Answer from the drawing. Dimensions are ordinates in mm from the lowest x, y and z of the part. A direction names the side the tool comes from. Give positions to 0.01 mm unless a question says otherwise; leave off trailing zeros. Write each loop counter-clockwise with the first axis right and the second up, starting at its lowest first coordinate (ties: lowest second). Pieces come first, ordered by that corner, then holes.
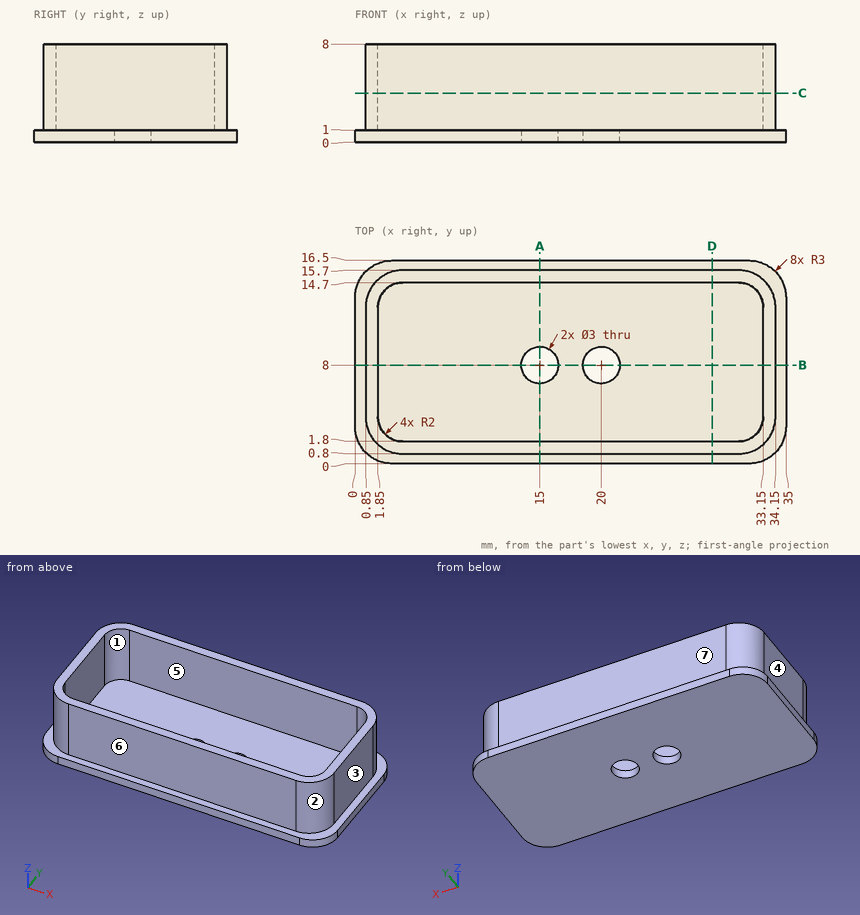
Item 1: Which of the six approach directions +Z, -Z, +X, -X, +Y, -Y give full straight-line access (tool end or side, diameter ignored) to the marked faces 4, 5, 6 and 7?
Result set:
face 4: +Z, -X, +Y, -Y
face 5: +Z
face 6: +Z, +X, -X, -Y
face 7: +Z, +X, -X, +Y
Item 2: Each of these flat-tipped pins is pushed along its axis until it touches: pin 1 Ø4 at (x, z) = (29, 7) entering from +Y; pin 2 Ø5 at (x, y) = (26.5, 10.5) entering from +Z; pin 3 Ø3.5 at (x, z) = (21.5, 4) entering from -Y; pin 4 Ø1.8 at (x, y) = (20, 8) entering from -Z. Where does it stop, or does it pass through?
Result set:
pin 1: stops at y = 15.7
pin 2: stops at z = 1
pin 3: stops at y = 0.8
pin 4: passes through
Item 3: Section A-A (x = 15) is taken. Write down the section's boundary in (y, z).
Result set:
outline: (0, 0) - (6.5, 0) - (6.5, 1) - (1.8, 1) - (1.8, 8) - (0.8, 8) - (0.8, 1) - (0, 1) - close; (9.5, 0) - (16.5, 0) - (16.5, 1) - (15.7, 1) - (15.7, 8) - (14.7, 8) - (14.7, 1) - (9.5, 1) - close
Item 4: Find the intervals of material crossed by line 1 along X through (y, z) = (8, 0.3); line 2 along Y through (x, z) = (20, 0.5); line 3 along Y through (x, z) = (6, 5), in increasing order.
Result set:
line 1: x = 0 to 13.5, 16.5 to 18.5, 21.5 to 35
line 2: y = 0 to 6.5, 9.5 to 16.5
line 3: y = 0.8 to 1.8, 14.7 to 15.7
Item 5: Section B-B (y = 8) is taken. Write down the section's boundary in (x, z).
Result set:
outline: (0, 0) - (13.5, 0) - (13.5, 1) - (1.85, 1) - (1.85, 8) - (0.85, 8) - (0.85, 1) - (0, 1) - close; (16.5, 0) - (18.5, 0) - (18.5, 1) - (16.5, 1) - close; (21.5, 0) - (35, 0) - (35, 1) - (34.15, 1) - (34.15, 8) - (33.15, 8) - (33.15, 1) - (21.5, 1) - close
Item 6: Section D-D (x = 29) is taken. Write down the section's boundary in (y, z), and give its area (3 significant figures).
Result set:
outline: (0, 0) - (16.5, 0) - (16.5, 1) - (15.7, 1) - (15.7, 8) - (14.7, 8) - (14.7, 1) - (1.8, 1) - (1.8, 8) - (0.8, 8) - (0.8, 1) - (0, 1) - close
area: 30.5 mm2
Item 7: Section C-C (z = 4) is taken. Write down the section's boundary in (x, y).
Result set:
outline: (0.85, 3.8) arc R3 ccw to (3.85, 0.8) - (31.15, 0.8) arc R3 ccw to (34.15, 3.8) - (34.15, 12.7) arc R3 ccw to (31.15, 15.7) - (3.85, 15.7) arc R3 ccw to (0.85, 12.7) - close; hole (1.85, 3.8) arc R2 ccw to (3.85, 1.8) - (31.15, 1.8) arc R2 ccw to (33.15, 3.8) - (33.15, 12.7) arc R2 ccw to (31.15, 14.7) - (3.85, 14.7) arc R2 ccw to (1.85, 12.7) - close
Item 8: Determine the mould class of the marked faces 1, 2 and 3 for opening direction Y: pulls with the +Y half, pulls with the -Y half, needs draft (parallel to the pull), parting line crosses it, or undercut.
Result set:
face 1: undercut
face 2: pulls with the -Y half
face 3: needs draft
